Design review of the part built by this model. Coordinates are the model's own, in mm. Face numbers are marked on the shaded views. A direction names the side the tool comes from. Coordinates: 2 decimals unless noted, no trailing zeros. Write each loop counter-clockwise with the first axis right and the second up, starting at its lowest first coordinate (ties: lowest second). Pieces come first, ordered by that corner, then holes.
Q1. Add section D-D, the plane y = 2.5. Give the boundary of the cut face in (x, z).
Q2. Clearance check with flat-ended pins moving along their axes: pin 1 Ø1.2 at (x, z) = (1, 18.5) entering from -Y; pin 2 Ø2.5 at (x, y) = (-11, 0) entering from -Z. State where each tip first meets the part, or that it passes through.
Q3. Add section C-C, the plane z = 19.25. Give the boundary of the cut face in (x, y).
Q4. Add section A-A, the plane x = 0. Give the boundary of the cut face in (y, z), plus the area to 3 significant figures.
Q5. To check wall thickness, follow probe 1 along X at (y, z) = (0, 18.25); probe 2 along Y at (x, z) = (-8.25, 15.25); probe 3 along X at (y, z) = (-0.75, 17). State the ranges of each line that lie inside material, in increasing order.
Q6. Add section B-B, the plane y = -0.5. Give the boundary of the cut face in (x, z), plus the area to 3 significant figures.
Q7. Machinability: for the marked faces 1, 2, 3 and 4, which of the approach directions +Z, -Z, +X, -X, +Y, -Y give a long, thin tool a straight path to every point of the face, cutting with its end or side? Answer none if there is none.
Q8. The part is to be moulded in two halves that separate along Y. For the marked faces 5, 6 and 7, say which applies: +Y half, -Y half, draft (parallel to the pull), parting line (faces both ways), or undercut.
Autodesk Inventor part; units mm, degrees
ref_plane "YZ Plane" through (0, 0, 0) normal (1, 0, 0) x (0, 1, 0)
ref_plane "XZ Plane" through (0, 0, 0) normal (0, 1, 0) x (-1, 0, 0)
ref_plane "XY Plane" through (0, 0, 0) normal (0, 0, 1) x (1, 0, 0)
sketch "スケッチ1" plane through (0, 0, 0) normal (0, 0, 1) x (1, 0, 0)
  line L0 (12, -3) -> (-12, -3)
  line L1 (-12, -3) -> (-12, 3)
  line L2 (-12, 3) -> (12, 3)
  line L3 (12, 3) -> (12, -3)
  line L4 (12, -3) -> (-12, 3) construction
  line L5 (-12, -3) -> (12, 3) construction
  point P0 (0, 0)
  dimension "d0" = 24
  dimension "d1" = 6
extrude "押し出し1" add sketch "スケッチ1" along normal blind 20
sketch "スケッチ2" plane through (-12, -3, 0) normal (0, -1, 0) x (1, 0, 0)
  line L0 (23.1845, 35.5) -> (0.8155, 35.5)
  arc A0 (0.8155, 35.5) -> (-4.2691, 17.077) centre (12, 22.5) ccw
  arc A1 (-4.2691, 17.077) -> (0, 14) centre (0, 18.5) ccw
  line L1 (0, 14) -> (0, 17)
  arc A2 (0, 20) -> (0, 17) centre (0, 18.5) ccw
  line L2 (0, 20) -> (3.2964, 20)
  arc A3 (4.3735, 20) -> (3.2964, 20) centre (3.8349, 18.6) ccw
  line L3 (4.3735, 20) -> (7.6699, 20)
  arc A4 (16.3301, 20) -> (7.6699, 20) centre (12, 22.5) ccw
  line L4 (16.3301, 20) -> (19.6265, 20)
  arc A5 (20.7036, 20) -> (19.6265, 20) centre (20.1651, 18.6) ccw
  line L5 (20.7036, 20) -> (24, 20)
  arc A6 (24, 17) -> (24, 20) centre (24, 18.5) ccw
  line L6 (24, 17) -> (24, 14)
  arc A7 (24, 14) -> (28.2691, 17.077) centre (24, 18.5) ccw
  arc A8 (28.2691, 17.077) -> (23.1845, 35.5) centre (12, 22.5) ccw
  circle A9 centre (25, 24.5) radius 1.6
  circle A10 centre (12, 32.5) radius 1.6
  circle A11 centre (-1, 24.5) radius 1.6
  line L7 (24, 0) -> (0, 0)
  line L8 (24, 0) -> (24, 14)
  line L9 (0, 20) -> (24, 20)
  circle A12 centre (12, 12.5) radius 1.6
  arc A13 (7.0148, 12.6154) -> (16.9852, 12.6154) centre (12, 13) ccw
  line L10 (3.8349, 18.6) -> (3.8349, 14) construction
  line L11 (20.1651, 18.6) -> (20.1651, 14) construction
  line L12 (0, 14) -> (5.5193, 14)
  line L13 (18.4807, 14) -> (24, 14)
  arc A14 (4.3735, 14) -> (3.2964, 14) centre (3.8349, 12.6) ccw
  arc A15 (20.7036, 14) -> (19.6265, 14) centre (20.1651, 12.6) ccw
  line L14 (5.3349, 18.6) -> (5.3349, 14) construction
  line L15 (18.6651, 18.6) -> (18.6651, 14) construction
  arc A16 (7.0148, 12.6154) -> (5.5193, 14) centre (5.5193, 12.5) ccw
  arc A17 (18.4807, 14) -> (16.9852, 12.6154) centre (18.4807, 12.5) ccw
  line L16 (0, 0) -> (0, 14)
  point P0 (12, 0)
  point P1 (7.101, 14)
  point P2 (16.899, 14)
  point P3 (12, 8)
  dimension "d5" = 3.2
  dimension "d6" = 10
  dimension "d7" = 4.5
  dimension "d8" = 5
  dimension "d11" = 3
  dimension "d12" = 3
  dimension "d13" = 1.4
  dimension "d14" = 1.5
  dimension "d15" = 1.5
  dimension "d16" = 1.5
extrude "押し出し2" cut sketch "スケッチ2" against normal through all contours L8 L7 L16 L12 A16 A13 A17 L13 | L13 A15 | A14 L12 | A12
sketch "スケッチ3" plane through (-12, -3, 20) normal (0, -1, 0) x (1, 0, 0)
  arc A0 (16.3301, 0) -> (7.6699, 0) centre (12, 2.5) ccw
  circle A1 centre (12, 2.5) radius 5
  point P0 (12, -20)
  dimension "d19" = 10
extrude "押し出し3" cut sketch "スケッチ3" against normal blind 2
sketch "スケッチ4" plane through (0, 0, 20) normal (0, 0, 1) x (1, 0, 0)
  circle A0 centre (8.1651, 0) radius 1.2295
  circle A1 centre (-8.1651, 0) radius 1.2295
  line L0 (-11.1845, 3) -> (11.1845, 3)
  line L1 (-11.1845, -3) -> (-11.1845, 3)
  line L2 (11.1845, -3) -> (-11.1845, -3)
  line L3 (11.1845, 3) -> (11.1845, -3)
  point P0 (0, 0)
hole "穴1" at (-8.1651, 0, 20) at (8.1651, 0, 20) direction (0, 0, -1) diameter 3.2 end through all
properties part number "DfixPit"
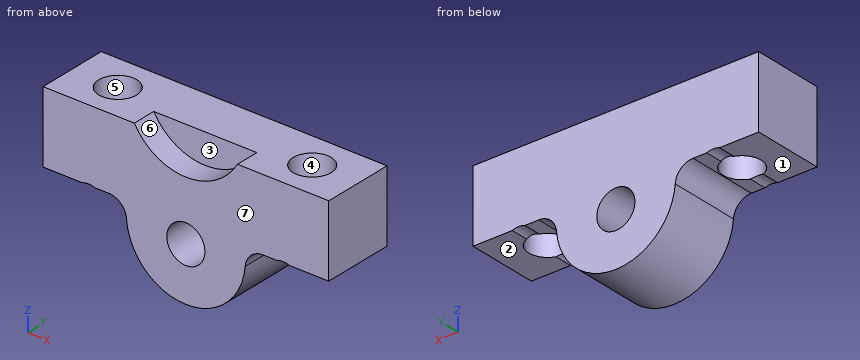
Here are the results:
1. outline: (-12, 14) - (-8.7, 14) arc R1.5 cw to (-7.63, 14) - (-6.48, 14) arc R1.5 cw to (-4.99, 12.62) arc R5 ccw to (4.99, 12.62) arc R1.5 cw to (6.48, 14) - (7.63, 14) arc R1.5 cw to (8.7, 14) - (12, 14) - (12, 20) - (-12, 20) - close; hole circle Ø3.2 at (0, 12.5)
2. pin 1: stops at y = -1
2. pin 2: stops at z = 14
3. outline: (-12, -3) - (-3.8, -3) - (-3.8, -1) - (3.8, -1) - (3.8, -3) - (12, -3) - (12, 3) - (-12, 3) - close; hole circle Ø3.2 at (-8.17, 0); hole circle Ø3.2 at (8.17, 0)
4. outline: (-3, 8) - (3, 8) - (3, 10.9) - (-3, 10.9) - close; (-3, 14.1) - (3, 14.1) - (3, 20) - (-1, 20) - (-1, 17.5) - (-3, 17.5) - close
4. area: 47.8 mm2
5. probe 1: x = -12 to -9.77, -6.57 to 6.57, 9.77 to 12
5. probe 2: y = -3 to -1.6, 1.6 to 3
5. probe 3: x = -12 to -9.58, -6.75 to 6.75, 9.58 to 12
6. outline: (-12, 14) - (-9.68, 14) - (-9.68, 20) - (-12, 20) - close; (-6.65, 14) - (-6.48, 14) arc R1.5 cw to (-4.99, 12.62) arc R5 ccw to (4.99, 12.62) arc R1.5 cw to (6.48, 14) - (6.65, 14) - (6.65, 20) - (-6.65, 20) - close; (9.68, 14) - (12, 14) - (12, 20) - (9.68, 20) - close; hole circle Ø3.2 at (0, 12.5)
6. area: 150 mm2
7. face 1: -Z, -X, +Y, -Y
7. face 2: -Z, +X, +Y, -Y
7. face 3: +Z, -Y
7. face 4: +Z, -Z
8. face 5: undercut
8. face 6: draft
8. face 7: -Y half
